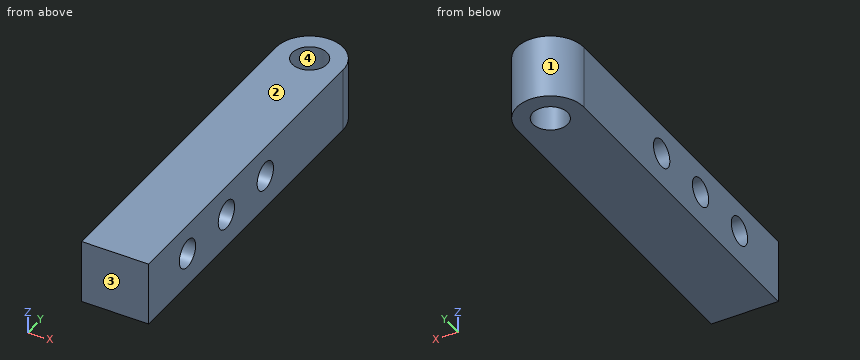
```python
from build123d import *

# Parameters (mm, degrees)
SKETCH_1_R          = 2.6
EXTRUDE_1_DEPTH     = 9.5
SKETCH_2_R          = 2.1
CUT_EXTRUDE_1_DEPTH = 10


with BuildPart() as part:
    # 草图1 → 凸台-拉伸1 (new body)
    with BuildSketch(Plane.XY):
        with BuildLine():
            Line((-5, 0), (-5, -50))
            Line((-5, -50), (5, -50))
            Line((5, -50), (5, 0))
            ThreePointArc((5, 0), (0, 5), (-5, 0))
        make_face()
        Circle(SKETCH_1_R, mode=Mode.SUBTRACT)
    extrude(amount=EXTRUDE_1_DEPTH)

    # 草图2 → 切除-拉伸1 (cut)
    with BuildSketch(Plane.ZY.offset(5)):
        with Locations(Location((5, -20, 0), (0, 0, 270))):
            Circle(SKETCH_2_R)
        with Locations(Location((5, -30, 0), (0, 0, 270))):
            Circle(SKETCH_2_R)
        with Locations(Location((5, -40, 0), (0, 0, 270))):
            Circle(SKETCH_2_R)
    extrude(amount=-CUT_EXTRUDE_1_DEPTH, mode=Mode.SUBTRACT)


solid = part.part
```
Source: CAD feature listing. Evaluate the final solid. Frame: model axes, mm. Face numbers are marked on the shaded views. Round coordinates to 2 decimals unless told otherwise and drop trailing zeros. Write each loop counter-clockwise with the first axis right and the second up, starting at its lowest first coordinate (ties: lowest second). Pieces come first, ordered by that corner, then holes. Notation, with made-up numbers: M 45.25,41 L 100.25,41 A18 ccw 100.25,70 Z; hole C 65,83 d4. An arc over 180 degrees is marked long. Answer as a JSON object with one key per item and string values. Group by question number.
(1) First-contact query: pin 1 (2.5 mm diameter, centred on y = -30, z = 5, fed in from +X). Flat tip, straight axial feed; report the tip coordinate or a pass-through.
(2) Section query A-A on x = 0. Output: boundary loops of the cut face in (y, z), then the cut area to 3 significant figures.
(3) Mould query, pull axis Y, two halves, no side actions, for the marked faces 1, 2, 3 and 4. Classes: +Y half, -Y half, draft (parallel to the pull), parting line (faces both ways), or undercut.
(4) Section query B-B on y = -30. Output: boundary loops of the cut face in (x, z), then the cut area to 3 significant figures.
(5) Section query D-D on z = 8.25. Output: boundary loops of the cut face in (x, y), then the cut area to 3 significant figures.
(6) Section query C-C on z = 6.25. Output: boundary loops of the cut face in (x, y), then the cut area to 3 significant figures.
(7) Ray query, line 1 (Z direction, x = -2.75, y = -40); line 2 (Y direction, x = 0.75, z = 5.75); line 3 (Y direction, x = 2, z = 5.5). Return the intervals inside material, ascending. Write a range as [from, to].
Computed values:
{
 "1": {"pin 1": "through"},
 "2": {"outline": "M -50,0 L -2.6,0 L -2.6,9.5 L -50,9.5 Z; M 2.6,0 L 5,0 L 5,9.5 L 2.6,9.5 Z; hole C -40,5 d4.2; hole C -30,5 d4.2; hole C -20,5 d4.2", "area": "432 mm^2"},
 "3": {"face 1": "+Y half", "face 2": "draft", "face 3": "-Y half", "face 4": "undercut"},
 "4": {"outline": "M -5,0 L 5,0 L 5,2.9 L -5,2.9 Z; M -5,7.1 L 5,7.1 L 5,9.5 L -5,9.5 Z", "area": "53.0 mm^2"},
 "5": {"outline": "M -5,-50 L 5,-50 L 5,0 A5 ccw -5,0 Z; hole C 0,0 d5.2", "area": "518 mm^2"},
 "6": {"outline": "M -5,-50 L 5,-50 L 5,-41.69 L -5,-41.69 Z; M -5,-38.31 L 5,-38.31 L 5,-31.69 L -5,-31.69 Z; M -5,-28.31 L 5,-28.31 L 5,-21.69 L -5,-21.69 Z; M -5,-18.31 L 5,-18.31 L 5,0 A5 ccw -5,0 Z; hole C 0,0 d5.2", "area": "417 mm^2"},
 "7": {"line 1": "[0, 2.9], [7.1, 9.5]", "line 2": "[-50, -41.96], [-38.04, -31.96], [-28.04, -21.96], [-18.04, -2.49], [2.49, 4.94]", "line 3": "[-50, -42.04], [-37.96, -32.04], [-27.96, -22.04], [-17.96, -1.66], [1.66, 4.58]"}
}
